Could you check a few things on this model? Use its own coordinates, in mm. Face numbers are marked on the shaded views. A direction names the side the tool comes from. Give positions to 0.01 mm unless a question says otherwise; leave off trailing zeros. Order: outer loops, then holes, each group sorted by start corner. A loop starts at its lowest first (then second) coordinate and runs counter-clockwise, first axis right, second up.
(1) On a 3-axis mill with a long thin cutter (end or side, diameter ignored), from which of +Z, -Z, +X, -X, +Y, -Y can I reach the whole of each face in a straight line? I mean the marked faces 1 and 2. Say none if no direction works.
(2) Imagine slicing it at A-A, the plane y = 165.5. Write out the boundary of the cut face in (x, z).
(3) If I drill on probe 1 along X at (y, z) = (4, 31); probe 2 along Y at (x, z) = (-154.5, 18.5); probe 3 along Y at (x, z) = (-235, 23), over which ranges is the centre line in solid material (lowest first)?
(4) Imagine slicing it at B-B, the plane x = -46. Write out the boundary of the cut face in (y, z), then the cut area to 3 significant figures.
(5) If we mould it in two halves opening along X, with no side actions, what happens to the marked faces 3, 4 and 5? For each: released by +X, released by -X, zero draft, split by the parting line, or undercut.
(6) Imagine slicing it at C-C, the plane z = 56. State how many separate pieces and enclosed holes the cut face has, then the cut area to 3 significant figures.
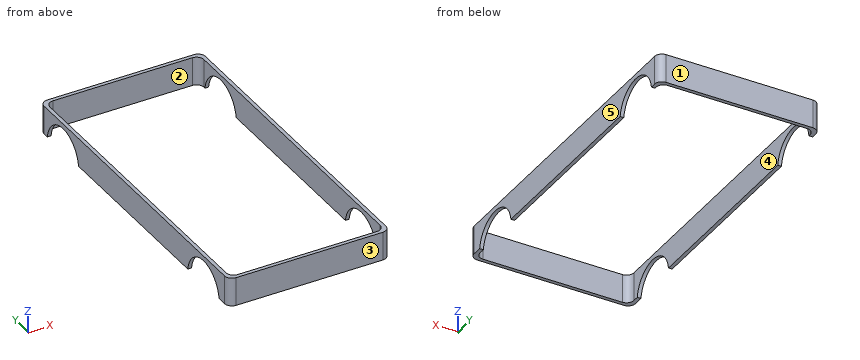
from build123d import *

# Parameters (mm, degrees)
SKETCH_1_W          = 440.4
SKETCH_1_H          = 900
SKETCH_1_W_2        = 420.4
SKETCH_1_H_2        = 880
EXTRUDE_1_DEPTH     = 78
FILLET_1_R          = 20
FILLET_2_R          = 20
CUT_EXTRUDE_1_DEPTH = 730
CUT_EXTRUDE_2_DEPTH = 730


with BuildPart() as part:
    # 草图1 → 凸台-拉伸1 (new body)
    with BuildSketch(Plane.XY):
        with Locations((-39.8, 0)):
            Rectangle(SKETCH_1_W, SKETCH_1_H)
        with Locations((-39.8, 0)):
            Rectangle(SKETCH_1_W_2, SKETCH_1_H_2, mode=Mode.SUBTRACT)
    extrude(amount=EXTRUDE_1_DEPTH)

    # 圆角1
    fillet_1_edges = [part.edges().sort_by_distance(p)[0] for p in [
        (180.4, -450, 39),
        (-260, -450, 39),
        (-260, 450, 39),
        (180.4, 450, 39),
    ]]
    fillet(fillet_1_edges, radius=FILLET_1_R)

    # 圆角2
    fillet_2_edges = [part.edges().sort_by_distance(p)[0] for p in [
        (170.4, -440, 39),
        (170.4, 440, 39),
        (-250, 440, 39),
        (-250, -440, 39),
    ]]
    fillet(fillet_2_edges, radius=FILLET_2_R)

    # 草图2 → 切除-拉伸1 (cut)
    with BuildSketch(Plane(origin=(180.4, 0, 0), x_dir=(0, 0, -1), z_dir=(1, 0, 0))):
        with BuildLine():
            Line((0, 265.819656263), (0, 414.480343737))
            ThreePointArc((0, 414.480343737), (-65, 340.15), (0, 265.819656263))
        make_face()
    extrude(amount=-CUT_EXTRUDE_1_DEPTH, mode=Mode.SUBTRACT)

    # 草图3 → 切除-拉伸2 (cut)
    with BuildSketch(Plane(origin=(180.4, 0, 0), x_dir=(0, 0, -1), z_dir=(1, 0, 0))):
        with BuildLine():
            Line((0, -403.470343737), (0, -254.809656263))
            ThreePointArc((0, -254.809656263), (-65, -329.14), (0, -403.470343737))
        make_face()
    extrude(amount=-CUT_EXTRUDE_2_DEPTH, mode=Mode.SUBTRACT)


solid = part.part
Answer block:
1. face 1: +Z, -Z, +X, -X, +Y
1. face 2: +Z, -Z
2. outline: (-260, 0) - (-250, 0) - (-250, 78) - (-260, 78) - close; (170.4, 0) - (180.4, 0) - (180.4, 78) - (170.4, 78) - close
3. probe 1: x = -260 to -250, 170.4 to 180.4
3. probe 2: y = -450 to -440, 440 to 450
3. probe 3: y = -450 to -439.36, 439.36 to 450
4. outline: (-450, 0) - (-440, 0) - (-440, 78) - (-450, 78) - close; (440, 0) - (450, 0) - (450, 78) - (440, 78) - close
4. area: 1,560 mm2
5. face 3: zero draft
5. face 4: undercut
5. face 5: released by +X
6. separate pieces: 4
6. enclosed holes: 0
6. area: 23,600 mm2
